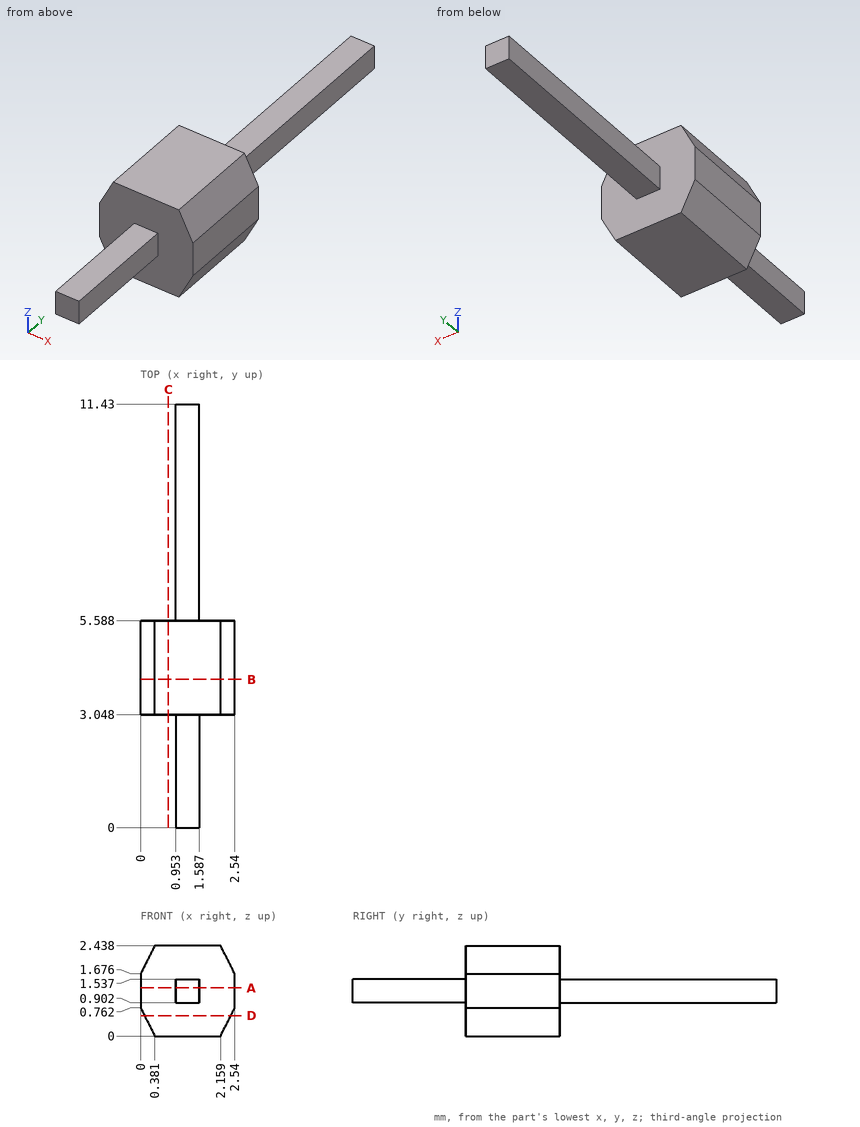
Print and shaded views of the part. All mm, measured from the part's lowest x, y and z. Coordinates: 2 decimals unless noted, no trailing zeros. Order: outer loops, then holes, each group sorted by start corner. A loop starts at its lowest first (then second) coordinate and runs counter-clockwise, first axis right, second up. Notation, with made-up numbers: M -32,40 L -1,40 A15 cw -1,65 Z; hole C 63,28 d5. An arc over 180 degrees is marked long. One line per question, with ' | ' between items. Start each with the question number.
Q1. Saw through at D-D (z = 0.55). List the corners of the cut face in (x, y) (1 decimal).
Q2. Saw through at B-B (y = 4). List the corners of the cut face in (x, z).
Q3. Saw through at A-A (z = 1.3). List the corners of the cut face in (x, y), then the cut area to 3 significant figures.
Q4. Saw through at C-C (x = 0.75). List the corners of the cut face in (y, z).
Q5. Probe L1, parallel to Z at x = 1.2, y = 2.5; L2, parallel to Y at x = 2.2, z = 1.9; L3, parallel to X at y = 7, z = 1.5. List the from-to ranges inside material, lowest first. Write a range as from..to.
Q6. Flat gauge pins, fed straight in: pin 1 Ø0.7 at (y, z) = (2, 1.5) entering from +X; pin 2 Ø0.7 at (x, y) = (1.5, 1) entering from -Z; pin 3 Ø1 at (x, y) = (0.5, 2.5) entering from +Z. Where does each tip first touch, or does it go through?
Check values:
1) outline: M 0.1,3 L 2.4,3 L 2.4,5.6 L 0.1,5.6 Z
2) outline: M 0,0.76 L 0.38,0 L 2.16,0 L 2.54,0.76 L 2.54,1.68 L 2.16,2.44 L 0.38,2.44 L 0,1.68 Z
3) outline: M 0,3.05 L 0.95,3.05 L 0.95,0 L 1.59,0 L 1.59,3.05 L 2.54,3.05 L 2.54,5.59 L 1.59,5.59 L 1.59,11.43 L 0.95,11.43 L 0.95,5.59 L 0,5.59 Z | area: 12.1 mm2
4) outline: M 3.05,0 L 5.59,0 L 5.59,2.44 L 3.05,2.44 Z
5) L1: z = 0.9..1.54 | L2: y = 3.05..5.59 | L3: x = 0.95..1.59
6) pin 1: stops at x = 1.59 | pin 2: stops at z = 0.9 | pin 3: stops at z = 1.54
